Input: part model. Units: mm. Frame: model coordinates. Face numbers are marked on the shaded views. A direction names the side the tool comes from. Round coordinates to 2 decimals unless told otherwise and drop trailing zeros. Order: outer loops, then holes, each group sorted by start corner. A loop starts at its lowest first (then second) coordinate and runs counter-clockwise, first axis right, second up.
Item 1: First-contact query: pin 1 (6 mm diameter, centred on x = -9, y = 38, fed in from -Z); pin 2 (6 mm diameter, centred on x = -8.5, z = 5.5, fed in from +Y); pin 3 (4.5 mm diameter, centred on x = -12, z = 5, fed in from -Y); pin 4 (3 mm diameter, centred on y = -48, z = 5, fed in from +X). Flat tips, straight axial feed; report the tip coordinate or a pass-through.
Item 2: Cut plane A-A on x = 0. Output: boundary loops of the cut face in (y, z).
Item 3: Line query: L1, parallel to Y at x = 0, z = 1.1; L2, parallel to Z at x = -13.15, y = 47.5; L3, parallel to Z at x = 7.75, y = 42. Output: solid intervals per line, ascending.
Item 4: Cut plane D-D on x = 11.5. Output: boundary loops of the cut face in (y, z).
Item 5: Cut plane C-C on y = 47.5. Output: boundary loops of the cut face in (x, z).
Item 6: Reachability of the marked faces 1 and 2 from +Z, -Z, +X, -X, +Y, -Y: full face, straight path, thin tool, end or side. Return the list, or none.
Item 7: Cut plane B-B on z = 7.5. Output: boundary loops of the cut face in (x, y), then the cut area to 3 significant figures.
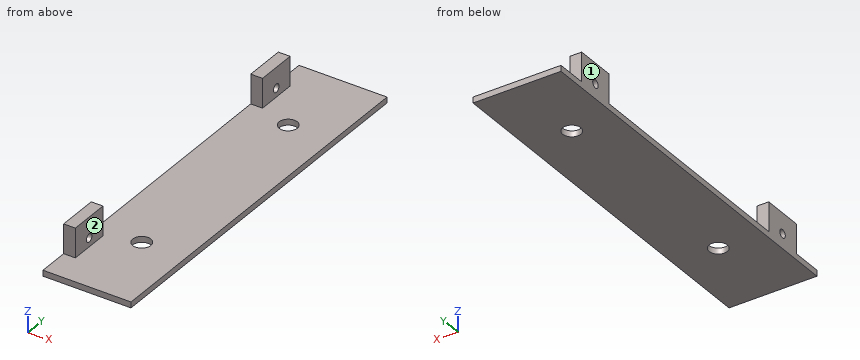
```python
from build123d import *

# Parameters (mm, degrees)
SKETCH_W     = 30
SKETCH_H     = 130
SKETCH_R     = 3.1
PAD_DEPTH    = 2
SKETCH001_W  = 4
SKETCH001_H  = 14
PAD001_DEPTH = 10
SKETCH002_R  = 1.4
POCKET_DEPTH = 5


with BuildPart() as part:
    # Sketch → Pad (new body)
    with BuildSketch(Plane.XY):
        Rectangle(SKETCH_W, SKETCH_H)
        with Locations((0, -37.18453)):
            Circle(SKETCH_R, mode=Mode.SUBTRACT)
        with Locations((0, 37.18453)):
            Circle(SKETCH_R, mode=Mode.SUBTRACT)
    extrude(amount=PAD_DEPTH)

    # Sketch001 (on Face8 of Pad) → Pad001 (join)
    with BuildSketch(Plane.XY.offset(2)):
        with Locations((-13, 47.5)):
            Rectangle(SKETCH001_W, SKETCH001_H)
        with Locations((-13, -47.5)):
            Rectangle(SKETCH001_W, SKETCH001_H)
    extrude(amount=PAD001_DEPTH)

    # Sketch002 (on Face7 of Pad001) → Pocket (cut)
    with BuildSketch(Plane(origin=(-15, 0, 0), x_dir=(0, -1, 0), z_dir=(-1, 0, 0))):
        with Locations((-47.5, 5)):
            Circle(SKETCH002_R)
        with Locations((47.5, 5)):
            Circle(SKETCH002_R)
    extrude(amount=-POCKET_DEPTH, mode=Mode.SUBTRACT)


solid = part.part
```
From the geometry:
1. pin 1: stops at z = 0
1. pin 2: stops at y = 54.5
1. pin 3: stops at y = -54.5
1. pin 4: stops at x = -11
2. outline: (-65, 0) - (-40.28, 0) - (-40.28, 2) - (-65, 2) - close; (-34.08, 0) - (34.08, 0) - (34.08, 2) - (-34.08, 2) - close; (40.28, 0) - (65, 0) - (65, 2) - (40.28, 2) - close
3. L1: y = -65 to -40.28, -34.08 to 34.08, 40.28 to 65
3. L2: z = 0 to 3.6, 6.4 to 12
3. L3: z = 0 to 2
4. outline: (-65, 0) - (65, 0) - (65, 2) - (-65, 2) - close
5. outline: (-15, 0) - (15, 0) - (15, 2) - (-11, 2) - (-11, 3.6) - (-15, 3.6) - close; (-15, 6.4) - (-11, 6.4) - (-11, 12) - (-15, 12) - close
6. face 1: +Z, -Z, -X, +Y, -Y
6. face 2: +Z, +X, +Y, -Y
7. outline: (-15, -54.5) - (-11, -54.5) - (-11, -40.5) - (-15, -40.5) - close; (-15, 40.5) - (-11, 40.5) - (-11, 54.5) - (-15, 54.5) - close
7. area: 112 mm2
